Source: CAD feature listing. Evaluate the final solid. Frame: model axes, mm. Give positions to 0.01 mm unless a question says otherwise; leave off trailing zeros. Loops run counter-clockwise (first coordinate to the right, second up) from the corner with the lowest first, then second, coordinate; pieces in that order, holes last.
```python
from build123d import *

# Parameters (mm, degrees)
BOSS_EXTRUDE1_DEPTH          = 3.175
F_6_CLEARANCE_HOLE1_D        = 4.3053
F_1_2_0_5_DIAMETER_HOLE1_D   = 12.7
F_1_8_0_125_DIAMETER_HOLE1_D = 3.175
CUT_EXTRUDE1_DEPTH           = 4.175
SKETCH10_W                   = 82.55
SKETCH10_H                   = 13.462
CUT_EXTRUDE2_DEPTH           = 4.175


with BuildPart() as part:
    # Sketch1 → Boss-Extrude1 (new body)
    with BuildSketch(Plane.XY):
        with BuildLine():
            Line((49.022, 13.462), (57.658, 13.462))
            ThreePointArc((57.658, 13.462), (61.250102448, 11.974102448), (62.738, 8.382))
            Line((62.738, 8.382), (62.738, 0))
            Line((62.738, 0), (82.55, 0))
            Line((82.55, 0), (82.55, 58.42))
            Line((82.55, 58.42), (0, 95.25))
            Line((0, 95.25), (0, 0))
            Line((0, 0), (43.942, 0))
            Line((43.942, 0), (43.942, 8.382))
            ThreePointArc((43.942, 8.382), (45.429897552, 11.974102448), (49.022, 13.462))
        make_face()
    extrude(amount=-BOSS_EXTRUDE1_DEPTH)

    # #6 Clearance Hole1 (through all)
    with Locations(Plane(origin=(0, 0, -3.175), x_dir=(-1, 0, 0), z_dir=(0, 0, -1))):
        with Locations((-4.8895, 17.4625), (-4.8895, 65.0875), (-76.2635, 36.5125), (-76.2635, 17.4625), (-28.194, 68.072), (-56.896, 30.48)):
            Hole(F_6_CLEARANCE_HOLE1_D / 2)

    # 1/2 (0.5) Diameter Hole1 (through all)
    with Locations(Plane(origin=(0, 0, -3.175), x_dir=(-1, 0, 0), z_dir=(0, 0, -1))):
        with Locations((-41.275, 46.99)):
            Hole(F_1_2_0_5_DIAMETER_HOLE1_D / 2)

    # 1/8 (0.125) Diameter Hole1 (through all)
    with Locations(Plane.XY):
        with Locations((41.275, 56.488873013)):
            Hole(F_1_8_0_125_DIAMETER_HOLE1_D / 2)

    # Sketch9 → Cut-Extrude1 (cut, through all)
    with BuildSketch(Plane.XY):
        Polygon((82.55, 56.681667019), (0, 93.511667019), (0, 95.25), (82.55, 58.42), align=None)
    extrude(amount=-CUT_EXTRUDE1_DEPTH, mode=Mode.SUBTRACT)

    # Sketch10 → Cut-Extrude2 (cut, through all)
    with BuildSketch(Plane.XY):
        with Locations((41.275, 6.731)):
            Rectangle(SKETCH10_W, SKETCH10_H)
    extrude(amount=-CUT_EXTRUDE2_DEPTH, mode=Mode.SUBTRACT)


solid = part.part
```
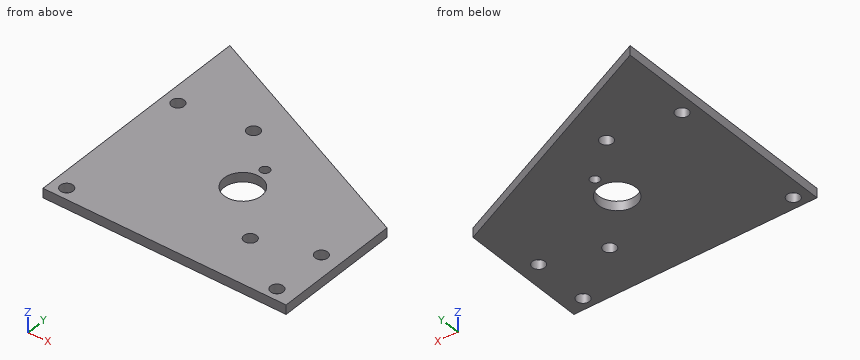
(1) First-contact query: pin 1 (5 mm diameter, centred on x = 28.194, y = 68.072, fed in from +Z). Flat tip, straight axial feed; report the tip coordinate or a pass-through.
A:
pin 1: stops at z = 0
(2) Section C-C, the plane x = 6. Return the cut outline in (y, z) (3 decimals), then the cut area to 3 significant figures.
A:
outline: (13.462, -3.175) - (15.618, -3.175) - (15.618, 0) - (13.462, 0) - close; (19.307, -3.175) - (63.243, -3.175) - (63.243, 0) - (19.307, 0) - close; (66.932, -3.175) - (90.835, -3.175) - (90.835, 0) - (66.932, 0) - close
area: 222 mm2
(3) Section A-A, the plane y = 46.99. Return the cut outline in (x, z) (3 decimals).
A:
outline: (0, -3.175) - (34.925, -3.175) - (34.925, 0) - (0, 0) - close; (47.625, -3.175) - (82.55, -3.175) - (82.55, 0) - (47.625, 0) - close
(4) Section D-D, the plane y = 30.48. Return the cut outline in (x, z) (3 decimals), then the cut area to 3 significant figures.
A:
outline: (0, -3.175) - (54.743, -3.175) - (54.743, 0) - (0, 0) - close; (59.049, -3.175) - (82.55, -3.175) - (82.55, 0) - (59.049, 0) - close
area: 248 mm2
(5) Section B-B, the plane z = -0.55. Count the separate pieces of the cut face and the enclosed holes in it, then the cut area to 3 significant figures.
A:
separate pieces: 1
enclosed holes: 8
area: 4,870 mm2
(6) Ray query, line 1 along Y through (x, z) = (76, -1.05); line 2 along X through (y, z) = (49.5, -2.45); line 3 along X through (y, z) = (42.5, -1.4). Return the intervals inside material, ascending.
A:
line 1: y = 13.46 to 15.33, 19.6 to 34.38, 38.65 to 59.6
line 2: x = 0 to 35.44, 47.11 to 82.55
line 3: x = 0 to 36.78, 45.77 to 82.55
